Source: three-view drawing plus pictorial views. Frame: mm from the lowest corner of the part. Coordinates: 2 decimals unless noted, no trailing zeros. Loops run counter-clockwise (first coordinate to the right, second up) from the corner with the lowest first, then second, coordinate; pieces in that order, holes last. Notation, with made-up numbers: (-27.75, 57) - (12.25, 57) arc R34 cw to (12.25, 93) - close; hole circle Ø7 at (-36, 70). An arc over 180 degrees is marked (long way). Return JSON: item names as keys, results as strings.
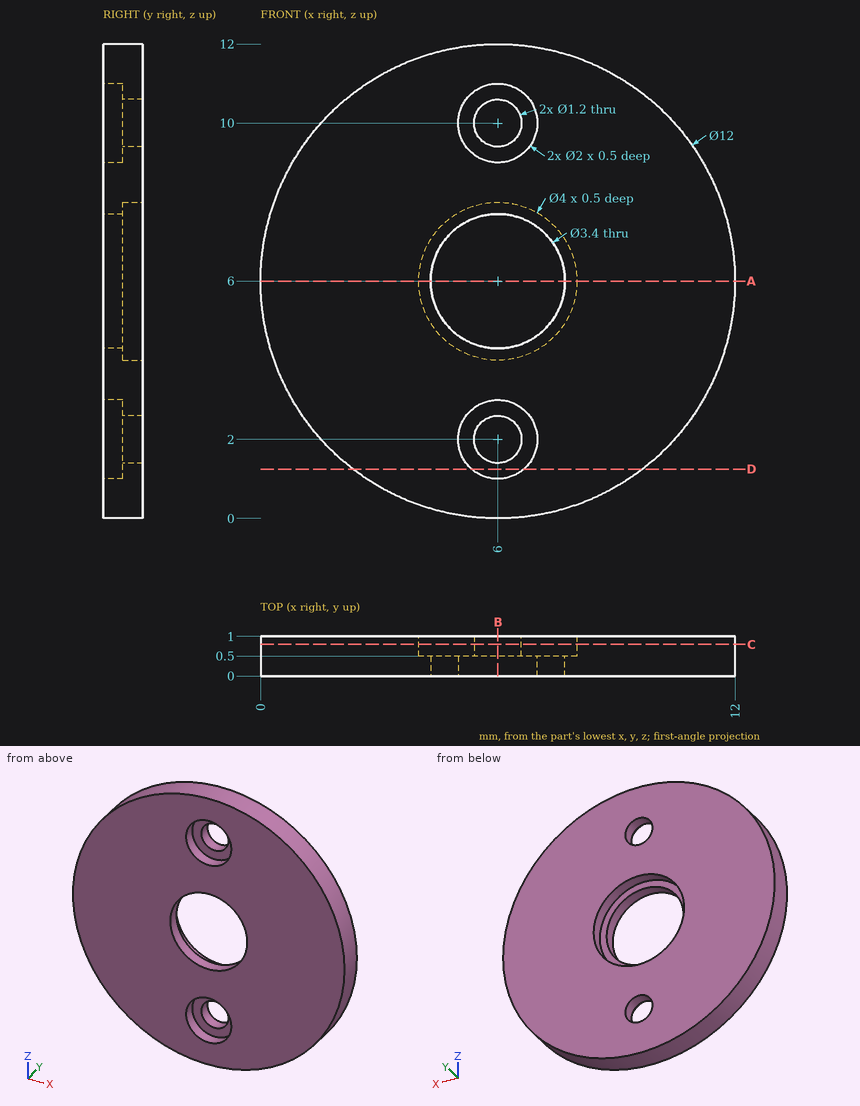
Item 1: Section query C-C, the plane y = 0.8. Return loops of the section in (x, z), and give its area (3 significant figures).
Worked out:
{"outline": "circle Ø12 at (6, 6); hole circle Ø4 at (6, 6); hole circle Ø1.2 at (6, 2); hole circle Ø1.2 at (6, 10)", "area": "98.3 mm^2"}
Item 2: Ray query, probe 1 along Z at (x, y) = (6, 0.95); probe 2 along Z at (x, y) = (6, 0.25); probe 3 along X at (y, z) = (0.2, 6). Return the intervals inside material, ascending. Write a range as from..to.
Worked out:
{"probe 1": "0..1.4, 2.6..4, 8..9.4, 10.6..12", "probe 2": "0..1, 3..4.3, 7.7..9, 11..12", "probe 3": "0..4.3, 7.7..12"}
Item 3: Section query A-A, the plane z = 6. Return loops of the section in (x, y), and give its area (3 significant figures).
Worked out:
{"outline": "(0, 0) - (4.3, 0) - (4.3, 0.5) - (4, 0.5) - (4, 1) - (0, 1) - close; (7.7, 0) - (12, 0) - (12, 1) - (8, 1) - (8, 0.5) - (7.7, 0.5) - close", "area": "8.30 mm^2"}
Item 4: First-contact query: pin 1 Ø0.6 at (x, z) = (6, 9.5) entering from -Y. Flat tip, straight axial feed; report the tip coordinate or a pass-through.
Worked out:
{"pin 1": "y = 0.5"}
Item 5: Section query D-D, the plane z = 1.25. Return loops of the section in (x, y), and give its area (3 significant figures).
Worked out:
{"outline": "(2.33, 0) - (5.34, 0) - (5.34, 0.5) - (6.66, 0.5) - (6.66, 0) - (9.67, 0) - (9.67, 1) - (2.33, 1) - close", "area": "6.67 mm^2"}
Item 6: Section query B-B, the plane x = 6. Return loops of the section in (y, z).
Worked out:
{"outline": "(0, 0) - (1, 0) - (1, 1.4) - (0.5, 1.4) - (0.5, 1) - (0, 1) - close; (0, 3) - (0.5, 3) - (0.5, 2.6) - (1, 2.6) - (1, 4) - (0.5, 4) - (0.5, 4.3) - (0, 4.3) - close; (0, 7.7) - (0.5, 7.7) - (0.5, 8) - (1, 8) - (1, 9.4) - (0.5, 9.4) - (0.5, 9) - (0, 9) - close; (0, 11) - (0.5, 11) - (0.5, 10.6) - (1, 10.6) - (1, 12) - (0, 12) - close"}
